```python
from build123d import *

# Parameters (mm, degrees)
SKETCH1_R                    = 17.5
SKETCH1_R_2                  = 15.9125
BOSS_EXTRUDE1_DEPTH          = 200
ESQUISSE1_R                  = 2.5
ENL_V_MAT_EXTRU_1_DEPTH      = 18.5
ENL_V_MAT_EXTRU_1_DEPTH_BACK = 18.5


with BuildPart() as part:
    # Sketch1 → Boss-Extrude1 (new body, symmetric)
    with BuildSketch(Plane.XY):
        Circle(SKETCH1_R)
        Circle(SKETCH1_R_2, mode=Mode.SUBTRACT)
    extrude(amount=BOSS_EXTRUDE1_DEPTH, both=True)

    # Esquisse1 → Enlèv. mat.-Extru.1 (cut, two sides)
    with BuildSketch(Plane(origin=(0, 0, 0), x_dir=(1, 0, 0), z_dir=(0, 1, 0))) as enl_v_mat_extru_1_sk:
        with Locations((0, 190)):
            Circle(ESQUISSE1_R)
        with Locations((0, -190)):
            Circle(ESQUISSE1_R)
    extrude(amount=ENL_V_MAT_EXTRU_1_DEPTH, mode=Mode.SUBTRACT)
    extrude(enl_v_mat_extru_1_sk.sketch, amount=-ENL_V_MAT_EXTRU_1_DEPTH_BACK, mode=Mode.SUBTRACT)


solid = part.part
```
Check sheet for the modelled part. Datum: model origin and axes. Units: mm. Give positions to 0.01 mm unless a question says otherwise; leave off trailing zeros. Loops run counter-clockwise (first coordinate to the right, second up) from the corner with the lowest first, then second, coordinate; pieces in that order, holes last. Notation, with made-up numbers: M 59.5,30.25 L 66.5,30.25 A22 cw 66.5,44.25 Z; hole C 68.25,28.25 d8. An arc over 180 degrees is marked long. Answer as CSV lines item,"result".
Item 1: Sectioned sample at C-C, the plane z = -104.5. Enter the section's corners in (x, y) (1 decimal).
Reply:
outline,"C 0,0 d35; hole C 0,0 d31.8"
Item 2: Scan lines: L1, parallel to Z at x = 0, y = 16; L2, parallel to Y at x = -3, z = -159; L3, parallel to Y at x = -1, z = 151. Record each from-to range of solid material in increasing order.
Reply:
L1,"-200 to -192.5, -187.5 to 187.5, 192.5 to 200"
L2,"-17.24 to -15.63, 15.63 to 17.24"
L3,"-17.47 to -15.88, 15.88 to 17.47"
Item 3: Depth check by flat-ended pin: pin 1 Ø4 at (x, z) = (-7.5, 154) entering from -Y; pin 2 Ø5 at (x, z) = (2, 43) entering from -Y; pin 3 Ø2 at (x, z) = (5, 47) entering from +Y; pin 4 Ø10 at (x, y) = (4, 6.5) entering from +Z. Enter the tip coordinate at first touch or a pass-through.
Reply:
pin 1,"y = -16.61"
pin 2,"y = -17.5"
pin 3,"y = 17.04"
pin 4,"through"
Item 4: Sectioned sample at A-A, the plane y = 0. Enter the section's corners in (x, z).
Reply:
outline,"M -17.5,-200 L -15.91,-200 L -15.91,200 L -17.5,200 Z; M 15.91,-200 L 17.5,-200 L 17.5,200 L 15.91,200 Z"
Item 5: Draft check along X on faces 1 (the face through (-13.887, -10.648, 2.8)), 2 (the face through (8, -14, 200)), 3 (the face through (-2.071, 15.777, -2.8)). Enter one of: pulls with the +X half, pulls with the -X half, needs draft (parallel to the pull), parting line crosses it, or undercut.
Reply:
face 1,"parting line crosses it"
face 2,"needs draft"
face 3,"undercut"
Item 6: Sectioned sample at B-B, the plane x = -7.5. Enter the section's corners in (y, z), then the cut area to 3 significant figures.
Reply:
outline,"M -15.81,-200 L -14.03,-200 L -14.03,200 L -15.81,200 Z; M 14.03,-200 L 15.81,-200 L 15.81,200 L 14.03,200 Z"
area,"1,420 mm^2"
